Autodesk Inventor part; units mm, degrees
ref_plane "YZ Plane" through (0, 0, 0) normal (1, 0, 0) x (0, 1, 0)
ref_plane "XZ Plane" through (0, 0, 0) normal (0, 1, 0) x (-1, 0, 0)
ref_plane "XY Plane" through (0, 0, 0) normal (0, 0, 1) x (1, 0, 0)
sketch "Skizze2" plane through (0, 0, 0) normal (0, 1, 0) x (-1, 0, 0)
  line L0 (-35, 0) -> (-35, -1075)
  line L1 (-35, -1075) -> (35, -1075)
  line L2 (35, -1075) -> (35, 0)
  line L3 (-25, 0) -> (-25, -1075)
  line L4 (-25, -1065) -> (25, -1065)
  line L5 (25, -1075) -> (25, 0)
  line L6 (0, 28) -> (0, -210) construction
  line L7 (35, 0) -> (25, 0)
  line L8 (-25, 0) -> (-35, 0)
  line L9 (25, -350) -> (-25, -350)
  line L10 (-25, -350) -> (-25, -360)
  line L11 (-25, -360) -> (25, -360)
  line L12 (25, -360) -> (25, -350)
  line L13 (25, -705) -> (-25, -705)
  line L14 (-25, -705) -> (-25, -715)
  line L15 (-25, -715) -> (25, -715)
  line L16 (25, -715) -> (25, -705)
  point P0 (0, 0)
  dimension "d0" = 70
  dimension "d1" = 10
  dimension "laenge" = 1075
  dimension "d3" = 10
  dimension "d4" = 35
  dimension "d6" = 10
  dimension "d7" = 350
  dimension "d8" = 10
  dimension "d9" = 705
extrude "Extrusion1" add sketch "Skizze2" along normal blind 10 contours L8 L3 L1 L0 | L3 L4 L5 L1 | L9 L5 L11 L3 | L5 L7 L2 L1 | L3 L13 L5 L15
sketch "Skizze3" plane through (0, 0, 0) normal (0, -1, 0) x (1, 0, 0)
  line L0 (25, -715) -> (-25, -715)
  line L1 (25, -1065) -> (25, -715)
  line L2 (-25, -1065) -> (25, -1065)
  line L3 (-25, -715) -> (-25, -1065)
  line L4 (35, -1075) -> (-35, -1075)
  line L5 (35, 0) -> (35, -1075)
  line L6 (25, 0) -> (35, 0)
  line L7 (25, -350) -> (25, 0)
  line L8 (-25, -350) -> (25, -350)
  line L9 (-25, 0) -> (-25, -350)
  line L10 (-35, 0) -> (-25, 0)
  line L11 (-35, -1075) -> (-35, 0)
  line L12 (-25, -360) -> (-25, -705)
  line L13 (25, -360) -> (-25, -360)
  line L14 (25, -705) -> (25, -360)
  line L15 (-25, -705) -> (25, -705)
  line L16 (-35, -1075) -> (-35, 0)
  line L17 (35, -1075) -> (-35, -1075)
  line L18 (-35, -1075) -> (-35, -335)
  line L19 (-35, -335) -> (35, -335)
  line L20 (35, -335) -> (35, -1075)
  circle A0 centre (-30, -1070) radius 1.5
  circle A1 centre (-30, -340) radius 1.5
  line L21 (-30, -340) -> (-30, -1070) construction
  circle A2 centre (-30, -578.3333) radius 1.5
  circle A3 centre (-30, -831.6667) radius 1.5
  line L22 (0, -209.5174) -> (0, -1351.6434) construction
  circle A4 centre (30, -1070) radius 1.5
  circle A5 centre (30, -340) radius 1.5
  circle A6 centre (30, -578.3333) radius 1.5
  circle A7 centre (30, -831.6667) radius 1.5
  point P0 (0, 0)
  dimension "abdeckung" = 740
  dimension "d13" = 3
  dimension "d14" = 5
  dimension "d15" = 5
  dimension "d16" = 3
  dimension "d17" = 5
  dimension "d19" = 5
  dimension "d20" = 3
  dimension "d21" = 243.3333
  dimension "d22" = 3
  dimension "d23" = 243.3333
properties part number "Makerbeam-Struktur" material "Aluminium 6061"
Verification items for the finished model (mm, model axes). Give positions to 0.01 mm unless a question says otherwise; leave off trailing zeros. Order: outer loops, then holes, each group sorted by start corner. A loop starts at its lowest first (then second) coordinate and runs counter-clockwise, first axis right, second up. Notation, with made-up numbers: (84.25, 59) - (126.25, 59) arc R26 cw to (126.25, 86) - close; hole circle Ø8 at (45.5, -37.75). An arc over 180 degrees is marked (long way). Answer as CSV lines item,"result". Start each with the question number.
Item 1: Section check C-C, the plane y = 6.25. Record the boundary of the cut face in (x, z), plus the area to 3 significant figures.
Item 2: Gauge pin test, flat end, axial feed: pin 1 (3 mm diameter, centred on x = 15, y = 6, fed in from +Z). Record the tip position at first contact, or that the pin passes through.
Item 3: Section check B-B, the plane x = -3.5. Record the boundary of the cut face in (y, z).
Item 4: Section check A-A, the plane z = -668. Record the boundary of the cut face in (x, y).
Item 5: Material ranges on L1, parallel to Z at x = -10, y = 7.75; L2, parallel to X at y = 7.25, z = -918.5, recorded low to high.
Filled in:
1,outline,"(-35, -1075) - (35, -1075) - (35, 0) - (25, 0) - (25, -350) - (-25, -350) - (-25, 0) - (-35, 0) - close; hole (-25, -1065) - (25, -1065) - (25, -715) - (-25, -715) - close; hole (-25, -705) - (25, -705) - (25, -360) - (-25, -360) - close"
1,area,"23,000 mm^2"
2,pin 1,"z = -350"
3,outline,"(0, -1075) - (10, -1075) - (10, -1065) - (0, -1065) - close; (0, -715) - (10, -715) - (10, -705) - (0, -705) - close; (0, -360) - (10, -360) - (10, -350) - (0, -350) - close"
4,outline,"(-35, 0) - (-25, 0) - (-25, 10) - (-35, 10) - close; (25, 0) - (35, 0) - (35, 10) - (25, 10) - close"
5,L1,"-1075 to -1065, -715 to -705, -360 to -350"
5,L2,"-35 to -25, 25 to 35"
